from build123d import *

# Parameters (mm, degrees)
SKETCH1_R          = 1.5
EXTRUDE1_DEPTH     = 4
SKETCH6_R          = 2.75
EXTRUDE2_DEPTH     = 3
CUT_EXTRUDE1_DEPTH = 1.875
CHAMFER1_SIZE      = 0.165


with BuildPart() as part:
    # Sketch1 → Extrude1 (new body)
    with BuildSketch(Plane.XY):
        Circle(SKETCH1_R)
    extrude(amount=-EXTRUDE1_DEPTH)

    # Sketch6 → Extrude2 (add)
    with BuildSketch(Plane(origin=(0, 0, -4), x_dir=(-1, 0, 0), z_dir=(0, 0, -1))):
        Circle(SKETCH6_R)
    extrude(amount=EXTRUDE2_DEPTH)

    # Sketch7 → Cut-Extrude1 (cut)
    with BuildSketch(Plane(origin=(0, 0, -7), x_dir=(-1, 0, 0), z_dir=(0, 0, -1))):
        Polygon((0, 1.443375673), (-1.25, 0.721687836), (-1.25, -0.721687836), (0, -1.443375673), (1.25, -0.721687836), (1.25, 0.721687836), align=None)
    extrude(amount=-CUT_EXTRUDE1_DEPTH, mode=Mode.SUBTRACT)

    # Cut-Extrude2 cone 1 section (through the dimple's axis) → Cut-Extrude2 (revolve, cut)
    with BuildSketch(Plane(origin=(0, 0, -7), x_dir=(0, 1, 0), z_dir=(1, 0, 0))):
        Polygon((0, 0), (1.443375673, 0), (0, 1.443375673), align=None)
    revolve(axis=Axis((0, 0, -7), (0, 0, 1)), mode=Mode.SUBTRACT)

    # Chamfer1
    chamfer1_edges = [part.edges().sort_by_distance(p)[0] for p in [
        (-1.5, 0, 0),
        (2.75, 0, -4),
        (2.75, 0, -7),
    ]]
    chamfer(chamfer1_edges, length=CHAMFER1_SIZE)


solid = part.part
Verification items for the finished model (mm, model axes). A direction names the side the tool comes from. Coordinates: 2 decimals unless noted, no trailing zeros. Loops run counter-clockwise (first coordinate to the right, second up) from the corner with the lowest first, then second, coordinate; pieces in that order, holes last. Notation, with made-up numbers: (36.25, 10) -> (52.25, 10) arc R22 cw to (52.25, 17) -> close; hole circle Ø1 at (28, 20.25). An arc over 180 degrees is marked (long way). Answer as a JSON object with one key per item and string values. Group by question number.
Item 1: Mould release check, pull along X, two halves, no side actions. Record for faces 4 (the cylindrical face through (0.596, -2.685, -5.481)), 5 (the flat face through (-2, 0, -4)), 6 (the flat face through (1.25, 0, -6)): +X half, -X half, draft (parallel to the pull), parting line (faces both ways), or undercut.
Item 2: Sectioned sample at C-C on z = -4.5. Record the boundary of the cut face in (x, y).
Item 3: Sectioned sample at D-D on z = -1.25. Record the boundary of the cut face in (x, y), plus the area to 3 significant figures.
Item 4: Tool access check on faces 1 (the cylindrical face through (-1.5, 0.07, -2.06)), 2 (the flat face through (-2, 0, -7)), 3 (the flat face through (-1.25, 0, -6)). Record the directions out of +Z, -Z, +X, -X, +Y, -Y that give a thin tool (end or side, any length) a straight path to the whole face; none if there is none.
Item 5: Scan lines: probe 1 along Z at (x, y) = (1.75, 0.35); probe 2 along Z at (x, y) = (0.8, -0.75) (3 decimals); probe 3 along X at (y, z) = (-0.55, -6.5). Record each from-to range of solid material in increasing order.
Item 6: Sectioned sample at B-B on y = 0. Record the boundary of the cut face in (x, z) (3 decimals), plus the area to 3 significant figures.
Item 7: Sectioned sample at A-A on z = -5.5. Record the boundary of the cut face in (x, y).
Evaluation:
{
 "1": {"face 4": "parting line", "face 5": "draft", "face 6": "undercut"},
 "2": {"outline": "circle Ø5.5 at (0, 0)"},
 "3": {"outline": "circle Ø3 at (0, 0)", "area": "7.07 mm²"},
 "4": {"face 1": "+Z", "face 2": "-Z, +X, -X, +Y, -Y", "face 3": "-Z"},
 "5": {"probe 1": "z = -7 to -4", "probe 2": "z = -5.125 to 0", "probe 3": "x = -2.69 to -1.25, 1.25 to 2.69"},
 "6": {"outline": "(-2.75, -6.835) -> (-2.585, -7) -> (-1.443, -7) -> (-1.25, -6.807) -> (-1.25, -5.125) -> (1.25, -5.125) -> (1.25, -6.807) -> (1.443, -7) -> (2.585, -7) -> (2.75, -6.835) -> (2.75, -4.165) -> (2.585, -4) -> (1.5, -4) -> (1.5, -0.165) -> (1.335, 0) -> (-1.335, 0) -> (-1.5, -0.165) -> (-1.5, -4) -> (-2.585, -4) -> (-2.75, -4.165) -> close", "area": "23.7 mm²"},
 "7": {"outline": "circle Ø5.5 at (0, 0); hole (-1.25, -0.72) -> (0, -1.44) -> (1.25, -0.72) -> (1.25, 0.72) -> (0, 1.44) -> (-1.25, 0.72) -> close"}
}
